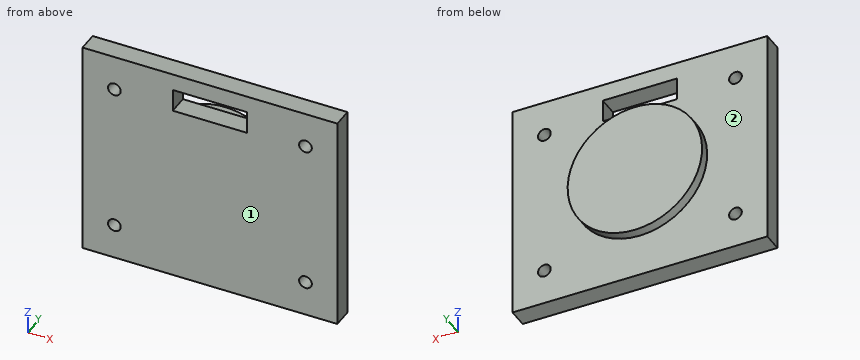
```python
from build123d import *

# Parameters (mm, degrees)
F_01_BASE_PROFILE_W           = 360
F_01_BASE_PROFILE_H           = 310
F_01_BASE_PROFILE_R           = 62.5
F_01_BASE_PROFILE_R_2         = 9
F_01_BASE_PROFILE_W_2         = 105
F_01_BASE_PROFILE_H_2         = 32
F_01_BASE_EXTRUDE_DEPTH       = 28
F_02_BOSS_PROFILE_R           = 95
F_02_REINFORCEMENT_BOSS_DEPTH = 42


with BuildPart() as part:
    # 01_Base_Profile → 01_Base_Extrude (new body)
    with BuildSketch(Plane(origin=(0, 0, 0), x_dir=(1, 0, 0), z_dir=(0, 1, 0))):
        Rectangle(F_01_BASE_PROFILE_W, F_01_BASE_PROFILE_H)
        with Locations(Location((0, 0, 0), (0, 0, 270))):
            Circle(F_01_BASE_PROFILE_R, mode=Mode.SUBTRACT)
        with Locations(Location((-135, -105, 0), (0, 0, 270))):
            Circle(F_01_BASE_PROFILE_R_2, mode=Mode.SUBTRACT)
        with Locations(Location((135, -105, 0), (0, 0, 270))):
            Circle(F_01_BASE_PROFILE_R_2, mode=Mode.SUBTRACT)
        with Locations(Location((-135, 105, 0), (0, 0, 270))):
            Circle(F_01_BASE_PROFILE_R_2, mode=Mode.SUBTRACT)
        with Locations(Location((135, 105, 0), (0, 0, 270))):
            Circle(F_01_BASE_PROFILE_R_2, mode=Mode.SUBTRACT)
        with Locations((0, -115)):
            Rectangle(F_01_BASE_PROFILE_W_2, F_01_BASE_PROFILE_H_2, mode=Mode.SUBTRACT)
    extrude(amount=F_01_BASE_EXTRUDE_DEPTH)

    # 02_Boss_Profile → 02_Reinforcement_Boss (add)
    with BuildSketch(Plane(origin=(0, 0, 0), x_dir=(1, 0, 0), z_dir=(0, 1, 0))):
        with Locations(Location((0, 0, 0), (0, 0, 90))):
            Circle(F_02_BOSS_PROFILE_R)
    extrude(amount=F_02_REINFORCEMENT_BOSS_DEPTH)


solid = part.part
```
For this review, take the finished solid that the model builds, in its own axes (mm). Face numbers are marked on the shaded views. A direction names the side the tool comes from. Coordinates: 2 decimals unless noted, no trailing zeros. Loops run counter-clockwise (first coordinate to the right, second up) from the corner with the lowest first, then second, coordinate; pieces in that order, holes last. Notation, with made-up numbers: (49.5, -28.75) -> (96.5, -28.75) arc R28 cw to (96.5, 9.25) -> close; hole circle Ø2 at (51, 49). An arc over 180 degrees is marked (long way). Return JSON: item names as keys, results as strings. Group by question number.
(1) Tool access review of the marked faces 1 and 2: name each direction out of +Z, -Z, +X, -X, +Y, -Y from which nothing blocks a thin tool from reaching the whole face with its end or side.
(2) Consider section D-D, the plane x = 57. Give the boundary of the cut face in (y, z), plus the area to 3 significant figures.
(3) To check wall thickness, follow L1, parallel to X at y = 11, z = 105; L2, parallel to X at y = 11.25, z = -105; L3, parallel to Z at x = 133.5, y = 21. State the ranges of each line that lie inside material, in increasing order.
(4) For pin 1 Ø11 at (x, z) = (-135, -105) entering from +Y; pin 2 Ø6 at (x, z) = (-133.5, 18.5) entering from +Y; pin 3 Ø6 at (x, y) = (-1.5, 32.5) entering from +Z, all flat-tipped, find the tip position at first contact; note any pin that passes through.
(5) Consider section B-B, the plane y = 16. Give the boundary of the cut face in (x, z).
(6) Consider section C-C, the plane z = 105. Give the boundary of the cut face in (x, y), plus the area to 3 significant figures.
(7) Consider section A-A, the plane z = -105. Give the boundary of the cut face in (x, y).
Results below:
{
 "1": {"face 1": "+Z, -Z, +X, -X, -Y", "face 2": "+Y"},
 "2": {"outline": "(0, -155) -> (28, -155) -> (28, -76) -> (42, -76) -> (42, 76) -> (28, 76) -> (28, 155) -> (0, 155) -> close", "area": "10,800 mm2"},
 "3": {"L1": "x = -180 to -144, -126 to -52.5, 52.5 to 126, 144 to 180", "L2": "x = -180 to -144, -126 to 126, 144 to 180", "L3": "z = -155 to -113.87, -96.13 to 96.13, 113.87 to 155"},
 "4": {"pin 1": "passes through", "pin 2": "stops at y = 28", "pin 3": "stops at z = 95"},
 "5": {"outline": "(-180, -155) -> (180, -155) -> (180, 155) -> (-180, 155) -> close; hole circle Ø18 at (-135, -105); hole circle Ø18 at (-135, 105); hole (-52.5, 99) -> (52.5, 99) -> (52.5, 131) -> (-52.5, 131) -> close; hole circle Ø18 at (135, -105); hole circle Ø18 at (135, 105)"},
 "6": {"outline": "(-180, 0) -> (-144, 0) -> (-144, 28) -> (-180, 28) -> close; (-126, 0) -> (-52.5, 0) -> (-52.5, 28) -> (-126, 28) -> close; (52.5, 0) -> (126, 0) -> (126, 28) -> (52.5, 28) -> close; (144, 0) -> (180, 0) -> (180, 28) -> (144, 28) -> close", "area": "6,130 mm2"},
 "7": {"outline": "(-180, 0) -> (-144, 0) -> (-144, 28) -> (-180, 28) -> close; (-126, 0) -> (126, 0) -> (126, 28) -> (-126, 28) -> close; (144, 0) -> (180, 0) -> (180, 28) -> (144, 28) -> close"}
}
